from build123d import *

# Parameters (mm, degrees)
SKETCH8_R           = 45
SKETCH8_R_2         = 2.65
BOSS_EXTRUDE4_DEPTH = 6
SKETCH9_R           = 1.65
CUT_EXTRUDE1_DEPTH  = 242.418521502
CUT_EXTRUDE2_DEPTH  = 242.418521502
FILLET2_R           = 10
FILLET3_R           = 5
SKETCH11_R          = 1.6
CUT_EXTRUDE3_DEPTH  = 242.418521502


with BuildPart() as part:
    # Sketch8 → Boss-Extrude4 (new body)
    with BuildSketch(Plane.XY):
        with BuildLine():
            Line((50, 177), (-50, 177))
            Line((-50, 177), (-147.758969873, 39.702478789))
            Line((-147.758969873, 39.702478789), (-147.758969873, 14.702478789))
            Line((-147.758969873, 14.702478789), (-25.330258141, -48.81985275))
            ThreePointArc((-25.330258141, -48.81985275), (2.348008246, -54.949857664), (29.402470247, -46.481122441))
            Line((29.402470247, -46.481122441), (164.066762399, 38.703198318))
            Line((164.066762399, 38.703198318), (164.066762399, 63.703198318))
            Line((164.066762399, 63.703198318), (50, 177))
        make_face()
        Circle(SKETCH8_R, mode=Mode.SUBTRACT)
        with Locations((-40, 169.5)):
            Circle(SKETCH8_R_2, mode=Mode.SUBTRACT)
        with Locations((40, 169.5)):
            Circle(SKETCH8_R_2, mode=Mode.SUBTRACT)
        with Locations((0, 169.5)):
            Circle(SKETCH8_R_2, mode=Mode.SUBTRACT)
        with Locations((40, 119.5)):
            Circle(SKETCH8_R_2, mode=Mode.SUBTRACT)
        with Locations((0, 119.5)):
            Circle(SKETCH8_R_2, mode=Mode.SUBTRACT)
        with Locations((-40, 119.5)):
            Circle(SKETCH8_R_2, mode=Mode.SUBTRACT)
    extrude(amount=BOSS_EXTRUDE4_DEPTH)

    # Sketch9 → Cut-Extrude1 (cut, through all)
    with BuildSketch(Plane(origin=(0, 0, 0), x_dir=(-1, 0, 0), z_dir=(0, 0, -1))):
        with Locations((35.355339059, -35.355339059)):
            Circle(SKETCH9_R)
        with Locations((-35.355339059, -35.355339059)):
            Circle(SKETCH9_R)
        with Locations((-35.355339059, 35.355339059)):
            Circle(SKETCH9_R)
        with Locations((35.355339059, 35.355339059)):
            Circle(SKETCH9_R)
    extrude(amount=-CUT_EXTRUDE1_DEPTH, mode=Mode.SUBTRACT)

    # Sketch10 → Cut-Extrude2 (cut, through all)
    with BuildSketch(Plane(origin=(0, 0, 0), x_dir=(-1, 0, 0), z_dir=(0, 0, -1))):
        with BuildLine():
            Line((45, 31.622776602), (45, 163.333195837))
            Line((45, 163.333195837), (138.48799676, 32.034040017))
            Line((138.48799676, 32.034040017), (54.193493342, 9.38431028))
            ThreePointArc((54.193493342, 9.38431028), (50.827892209, 21.012505171), (45, 31.622776602))
        make_face()
        with BuildLine():
            Line((-52.868310579, 15.163829877), (-154.461888015, 54.610185231))
            Line((-154.461888015, 54.610185231), (-45, 163.333195837))
            Line((-45, 163.333195837), (-45, 31.622776602))
            ThreePointArc((-45, 31.622776602), (-49.621323901, 23.721808833), (-52.868310579, 15.163829877))
        make_face()
    extrude(amount=-CUT_EXTRUDE2_DEPTH, mode=Mode.SUBTRACT)

    # Fillet2
    fillet2_edges = [part.edges().sort_by_distance(p)[0] for p in [
        (-54.193493342, 9.38431028, 3),
        (-45, 31.622776602, 3),
        (-45, 163.333195837, 3),
        (-138.48799676, 32.034040017, 3),
        (45, 31.622776602, 3),
        (52.868310579, 15.163829877, 3),
        (154.461888015, 54.610185231, 3),
        (45, 163.333195837, 3),
    ]]
    fillet(fillet2_edges, radius=FILLET2_R)

    # Fillet3
    fillet3_edges = [part.edges().sort_by_distance(p)[0] for p in [
        (-147.758969873, 39.702478789, 3),
        (-50, 177, 3),
        (50, 177, 3),
        (164.066762399, 63.703198318, 3),
        (164.066762399, 38.703198318, 3),
        (-147.758969873, 14.702478789, 3),
    ]]
    fillet(fillet3_edges, radius=FILLET3_R)

    # Sketch11 → Cut-Extrude3 (cut, through all)
    with BuildSketch(Plane(origin=(0, 0, 0), x_dir=(-1, 0, 0), z_dir=(0, 0, -1))):
        with Locations((142.758969873, 38.104287644)):
            Circle(SKETCH11_R)
        with Locations((142.758969873, 17.741175158)):
            Circle(SKETCH11_R)
        with Locations((-159.066762399, 61.622204822)):
            Circle(SKETCH11_R)
        with Locations((-159.066762399, 41.456738724)):
            Circle(SKETCH11_R)
    extrude(amount=-CUT_EXTRUDE3_DEPTH, mode=Mode.SUBTRACT)


solid = part.part
Build history of the part. All positions in model axes, mm. A direction names the side the tool comes from. Round coordinates to 2 decimals unless told otherwise and drop trailing zeros. Order: outer loops, then holes, each group sorted by start corner. A loop starts at its lowest first (then second) coordinate and runs counter-clockwise, first axis right, second up. Notation, with made-up numbers: M 17.5,24.5 L 72.5,24.5 A17 cw 72.5,37.5 Z; hole C 4.25,-29 d8. An arc over 180 degrees is marked long. Use CSV: the item, a comma, the result in double quotes. Start each with the question number.
(1) Cut at B-B on y = 0. List the corners of the cut face in (x, z).
(2) Tool access for faces 4 (the face through (55.024, 18.781, 3.042)), 5 (the face through (164.067, 51, 3)): list every direction of +Z, -Z, +X, -X, +Y, -Y with a clear straight run to the whole face (end or side of a thin tool).
(3) Cut at D-D on y = 156. List the corners of the cut face in (x, z).
(4) Drill centre lines: probe 1 along Y at (x, z) = (0, 3.55); probe 2 along X at (y, z) = (169.5, 1.65); probe 3 along Y at (x, z) = (40, 1.55). Where is each one in solid material? Low to high.
(5) Cut at C-C on z = 4.5. State how many separate pieces and enclosed holes the cut face has, then the cut area to 3 significant figures.
(6) Flat gauge pins, fed straight in: P1, Ø3, axis at y = 39, z = 3.5, coming from the +X side; P2, Ø1.5, axis at x = 66, z = 0.5, coming from the -Y side; P3, Ø1.8, axis at y = 79, z = 1.5, coming from the -X side. Where does each tip first touch, or does it go through?
(7) Cut at A-A on x = -10. List the corners of the cut face in (y, z), then the cut area to 3 significant figures.
(8) Mould opens along Y. For faces 1 (the face through (45, 88, 3)), 2 (the face through (-147.759, 28, 3)), 3 (the face through (107.8, 119.59, 2.96)) say: +Y half, -Y half, draft (parallel to the pull), parting line (faces both ways), or undercut.
Findings:
1,outline,"M -119.42,0 L -45,0 L -45,6 L -119.42,6 Z; M 45,0 L 102.88,0 L 102.88,6 L 45,6 Z"
2,face 4,"+Z, -Z"
2,face 5,"+Z, -Z, +X, +Y, -Y"
3,outline,"M -64.95,0 L 71.14,0 L 71.14,6 L -64.95,6 Z"
4,probe 1,"y = -55 to -45, 45 to 116.85, 122.15 to 166.85, 172.15 to 177"
4,probe 2,"x = -55.34 to -42.65, -37.35 to -2.65, 2.65 to 37.35, 42.65 to 57.55"
4,probe 3,"y = -39.78 to -20.62, 20.62 to 116.85, 122.15 to 166.85, 172.15 to 177"
5,separate pieces,"1"
5,enclosed holes,"17"
5,area,"26,000 mm^2"
6,P1,"stops at x = 163.97"
6,P2,"stops at y = -23.81"
6,P3,"stops at x = -120.42"
7,outline,"M -54.08,0 L -43.87,0 L -43.87,6 L -54.08,6 Z; M 43.87,0 L 177,0 L 177,6 L 43.87,6 Z"
7,area,"860 mm^2"
8,face 1,"undercut"
8,face 2,"draft"
8,face 3,"+Y half"
